Part model, mm, in its own coordinate system. Face numbers are marked on the shaded views. A direction names the side the tool comes from. Coordinates: 2 decimals unless noted, no trailing zeros. Order: outer loops, then holes, each group sorted by start corner. A loop starts at its lowest first (then second) coordinate and runs counter-clockwise, first axis right, second up.
1) Cut at C-C (y = 0.25). List the corners of the cut face in (x, z), and give its area (3 significant figures).
2) Pin check, flat tips, straight feed: pin 1 Ø4 at (x, z) = (-7, 13.5) entering from +Y; pin 2 Ø5 at (x, z) = (0, 15) entering from +Y; pin 3 Ø8 at (x, z) = (-7, 13.5) entering from -Y; pin 4 Ø6 at (x, y) = (0, 7) entering from -Z. Stop position of each tip, or through.
3) Cut at B-B (z = 28). List the corners of the cut face in (x, y).
4) Cut at A-A (x = 4.5). List the corners of the cut face in (y, z), and give its area (3 significant figures).
5) Cut at D-D (x = -7.5). List the corners of the cut face in (y, z), and give its area (3 significant figures).
6) Wall check: L1, parallel to Y at x = 0.75, z = 19; L2, parallel to Z at x = 1.5, y = 4.5. Give the ranges that are in metal, low to high.
7) Tool access for the marked faces 1 and 2: list every direction of +Z, -Z, +X, -X, +Y, -Y with a clear straight run to the whole face (end or side of a thin tool).
```python
from build123d import *

# Parameters (mm, degrees)
F2_DEPTH      = 1
F3_R          = 4
F4_W          = 18
F4_H          = 1
F5_DEPTH      = 1
F5_DEPTH_BACK = 10


with BuildPart() as f2:
    # F1 (on Front) → F2 (new body)
    with BuildSketch(Plane.XZ):
        Polygon((9, 30), (-9, 30), (0, 0), align=None)
    extrude(amount=F2_DEPTH)

    # F3
    f3_edges = [f2.edges().sort_by_distance(p)[0] for p in [
        (0, -0.5, 0),
    ]]
    fillet(f3_edges, radius=F3_R)

    # F4 (on face) → F5 (join, two sides)
    with BuildSketch(Plane.XZ) as f5_sk:
        with Locations((0, 30.5)):
            Rectangle(F4_W, F4_H)
    extrude(amount=F5_DEPTH)
    extrude(f5_sk.sketch, amount=-F5_DEPTH_BACK)


solid = f2.part
```
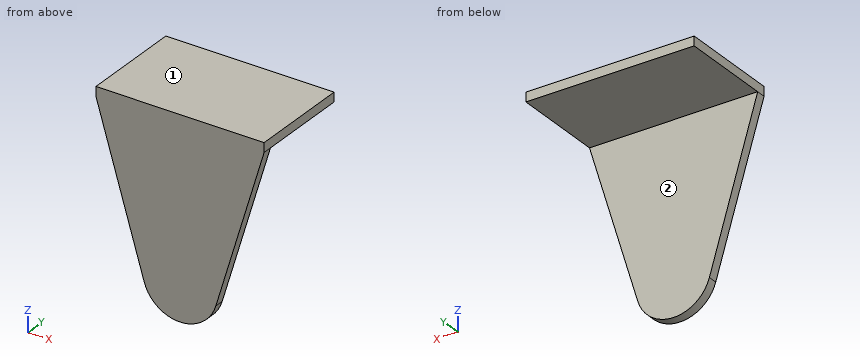
Geometry check:
1. outline: (-9, 30) - (9, 30) - (9, 31) - (-9, 31) - close
1. area: 18.0 mm2
2. pin 1: passes through
2. pin 2: stops at y = 0
2. pin 3: stops at y = -1
2. pin 4: stops at z = 30
3. outline: (-8.4, -1) - (8.4, -1) - (8.4, 0) - (-8.4, 0) - close
4. outline: (-1, 15) - (0, 15) - (0, 30) - (10, 30) - (10, 31) - (-1, 31) - close
4. area: 26.0 mm2
5. outline: (-1, 25) - (0, 25) - (0, 30) - (10, 30) - (10, 31) - (-1, 31) - close
5. area: 16.0 mm2
6. L1: y = -1 to 0
6. L2: z = 30 to 31
7. face 1: +Z, +X, -X, +Y, -Y
7. face 2: -Z, +X, -X, +Y
